For this review, take the finished solid that the model builds, in its own axes (mm). Give positions to 0.01 mm unless a question says otherwise; leave off trailing zeros. Loops run counter-clockwise (first coordinate to the right, second up) from the corner with the lowest first, then second, coordinate; pieces in that order, holes last. Notation, with made-up numbers: (60.5, 81) - (69.5, 81) arc R15 cw to (69.5, 90) - close; hole circle Ø1 at (60.5, 33). An arc over 180 degrees is marked (long way). Put each result on its own line as item: value. Start each with the question number.
from build123d import *

# Parameters (mm, degrees)
F0_W     = 76.2
F0_H     = 38.1
F0_W_2   = 4.3870395845
F0_H_2   = 20.68563866
F1_DEPTH = 12.7


with BuildPart() as f1:
    # F0 (on Top) → F1 (new body)
    with BuildSketch(Plane.XY):
        Rectangle(F0_W, F0_H)
        Polygon((-1.5570254376, -10.5457305908), (-6.2836191695, -10.5457305908), (-7.7821848067, -5.6199317591), (-15.3248142677, -5.6199317591), (-16.823379905, -10.5457305908), (-21.5499736369, -10.5457305908), (-14.2472957733, 10.2259284532), (-8.8868676329, 10.2259284532), align=None, mode=Mode.SUBTRACT)
        Polygon((13.8225137457, -10.5457305908), (1.0462230259, -10.5457305908), (1.0462230259, 10.1399080692), (5.4332626104, 10.1399080692), (5.4332626104, -6.9238196851), (13.8225137457, -6.9238196851), align=None, mode=Mode.SUBTRACT)
        with Locations((19.6107801118, -0.2029112608)):
            Rectangle(F0_W_2, F0_H_2, mode=Mode.SUBTRACT)
    extrude(amount=F1_DEPTH)


solid = f1.part
1) Mouldability with a two-part tool opening along Y and no side actions: class faces 1 (the flat face through (-38.1, 0, 6)), 2 (the flat face through (-1, -19.05, 6)), 3 (the flat face through (17.417, 0, 6)) as released by +Y, released by -Y, zero draft, split by the parting line, or undercut.
2) Take a section at A-A on x = 10.5. State the section outline as (y, z) points, and give its area (3 significant figures).
3) Take a section at D-D on x = -13.5. State the section outline as (y, z) points.
4) Take a section at C-C on z = 9.75. State the section outline as (x, y) points, and give its area (3 significant figures).
5) Wall thickness on probe 1 along Y at (x, z) = (-11.5, 1.75); probe 2 along Y at (x, z) = (10.5, 2.5); probe 3 along X at (y, z) = (-3, 2.5): over which ranges is each line inside the solid? List them lowest first.
6) Take a section at B-B on y = 4. State the section outline as (x, z) points, and give its area (3 significant figures).
Answers follow:
1. face 1: zero draft
1. face 2: released by -Y
1. face 3: undercut
2. outline: (-19.05, 0) - (-10.55, 0) - (-10.55, 12.7) - (-19.05, 12.7) - close; (-6.92, 0) - (19.05, 0) - (19.05, 12.7) - (-6.92, 12.7) - close
2. area: 438 mm2
3. outline: (-19.05, 0) - (-5.62, 0) - (-5.62, 12.7) - (-19.05, 12.7) - close; (10.23, 0) - (19.05, 0) - (19.05, 12.7) - (10.23, 12.7) - close
4. outline: (-38.1, -19.05) - (38.1, -19.05) - (38.1, 19.05) - (-38.1, 19.05) - close; hole (-21.55, -10.55) - (-16.82, -10.55) - (-15.32, -5.62) - (-7.78, -5.62) - (-6.28, -10.55) - (-1.56, -10.55) - (-8.89, 10.23) - (-14.25, 10.23) - close; hole (1.05, -10.55) - (13.82, -10.55) - (13.82, -6.92) - (5.43, -6.92) - (5.43, 10.14) - (1.05, 10.14) - close; hole (17.42, -10.55) - (21.8, -10.55) - (21.8, 10.14) - (17.42, 10.14) - close
4. area: 2,470 mm2
5. probe 1: -19.05 to -5.62, 10.23 to 19.05
5. probe 2: -19.05 to -10.55, -6.92 to 19.05
5. probe 3: -38.1 to -18.9, -4.22 to 1.05, 5.43 to 17.42, 21.8 to 38.1
6. outline: (-38.1, 0) - (-16.44, 0) - (-16.44, 12.7) - (-38.1, 12.7) - close; (-6.69, 0) - (1.05, 0) - (1.05, 12.7) - (-6.69, 12.7) - close; (5.43, 0) - (17.42, 0) - (17.42, 12.7) - (5.43, 12.7) - close; (21.8, 0) - (38.1, 0) - (38.1, 12.7) - (21.8, 12.7) - close
6. area: 733 mm2
